from build123d import *

# Parameters (mm, degrees)
BOSS_EXTRUDE1_DEPTH = 0.8
SKETCH2_W           = 0.45
SKETCH2_H           = 25.2222
BOSS_EXTRUDE2_DEPTH = 9.525


with BuildPart() as part:
    # Sketch1 → Boss-Extrude1 (new body)
    with BuildSketch(Plane.XY):
        Polygon((0, 0), (0, 25.2222), (6.1722, 25.2222), (6.1722, 15.6972), (15.6972, 15.6972), (15.6972, 9.525), (6.1722, 9.525), (6.1722, 0), align=None)
    extrude(amount=BOSS_EXTRUDE1_DEPTH)

    # Sketch2 → Boss-Extrude2 (add)
    with BuildSketch(Plane.XY.offset(0.8)):
        Polygon((6.1722, 0), (6.1722, 9.525), (15.6972, 9.525), (15.6972, 9.975), (5.7222, 9.975), (5.7222, 0), align=None)
        Polygon((15.6972, 15.6972), (6.1722, 15.6972), (6.1722, 25.2222), (5.7222, 25.2222), (5.7222, 15.2472), (15.6972, 15.2472), align=None)
        with Locations((0.225, 12.6111)):
            Rectangle(SKETCH2_W, SKETCH2_H)
    extrude(amount=BOSS_EXTRUDE2_DEPTH)


solid = part.part
The model under review builds one solid part; all positions refer to its coordinate system, in mm. A direction names the side the tool comes from. Round coordinates to 2 decimals unless told otherwise and drop trailing zeros. Loops run counter-clockwise (first coordinate to the right, second up) from the corner with the lowest first, then second, coordinate; pieces in that order, holes last. Notation, with made-up numbers: M -14.75,-31 L 30.25,-31 A28 cw 30.25,2 Z; hole C 38,74.25 d10. An arc over 180 degrees is marked long. Answer as CSV lines item,"result". Start each with the question number.
Item 1: Insertion check: P1, Ø4, axis at x = 12.5, z = 6.5, coming from the -Y side (3 decimals); P2, Ø1.5, axis at x = 11, z = 5, coming from the +Y side; P3, Ø2, axis at y = 4.5, z = 2, coming from the +X side; P4, Ø1, axis at x = 7, y = 3.5, coming from the +Z side. Each pin has a flat end and moves straight along its axis. Give the tip position at first contact, or say it passes through.
Item 2: Wall thickness on line 1 (X direction, y = 2, z = 6.25); line 2 (Y direction, x = 8, z = 1.5) (3 decimals); line 3 (X direction, y = 14, z = 1.25): over which ranges is each line inside the solid? List them lowest first. Write a range as [from, to].
Item 3: Consider section C-C (x = 10.5). Write out the cut boundary in (y, z) (3 decimals).
Item 4: For faces 5 (the face through (11, 15.697, 5)), 6 (the face through (11, 9.975, 5)), 7 (the face through (11, 9.525, 5)), 8 (the face through (5.722, 20, 5)), list the 3-axis set-ups (+Z, -Z, +X, -X, +Y, -Y) from which the entire face can be reached by the end or side of a thin tool; tool diameter is ignored.
Item 5: Consider section B-B (y = 21.75). Write out the cut boundary in (x, z) (3 decimals), then the cut area to 3 significant figures.
Item 6: Consider section A-A (z = 1.5). Write out the cut boundary in (x, y) (3 decimals).
Item 7: Consider section D-D (y = 10.5). Write out the cut boundary in (x, z) (3 decimals), then the cut area to 3 significant figures.
Item 8: Mouldability with a two-part tool opening along X and no side actions: class faces 1 (the face through (6.172, 5, 5)), 2 (the face through (0.3, 0, 3.6)), 3 (the face through (0.45, 12, 5)), 4 (the face through (5, 13, 0.8)) as released by +X, released by -X, zero draft, split by the parting line, or undercut.
Answer:
1,P1,"stops at y = 9.525"
1,P2,"stops at y = 15.7"
1,P3,"stops at x = 6.17"
1,P4,"passes through"
2,line 1,"x = [0, 0.45], [5.72, 6.17]"
2,line 2,"y = [9.525, 9.975], [15.247, 15.697]"
2,line 3,"x = [0, 0.45]"
3,outline,"M 9.525,0 L 15.697,0 L 15.697,10.325 L 15.247,10.325 L 15.247,0.8 L 9.975,0.8 L 9.975,10.325 L 9.525,10.325 Z"
4,face 5,"+Z, -Z, +X, +Y"
4,face 6,"+Z, +X"
4,face 7,"+Z, -Z, +X, -Y"
4,face 8,"+Z, +Y, -Y"
5,outline,"M 0,0 L 6.172,0 L 6.172,10.325 L 5.722,10.325 L 5.722,0.8 L 0.45,0.8 L 0.45,10.325 L 0,10.325 Z"
5,area,"13.5 mm^2"
6,outline,"M 0,0 L 0.45,0 L 0.45,25.222 L 0,25.222 Z; M 5.722,0 L 6.172,0 L 6.172,9.525 L 15.697,9.525 L 15.697,9.975 L 5.722,9.975 Z; M 5.722,15.247 L 15.697,15.247 L 15.697,15.697 L 6.172,15.697 L 6.172,25.222 L 5.722,25.222 Z"
7,outline,"M 0,0 L 15.697,0 L 15.697,0.8 L 0.45,0.8 L 0.45,10.325 L 0,10.325 Z"
7,area,"16.8 mm^2"
8,face 1,"released by +X"
8,face 2,"zero draft"
8,face 3,"undercut"
8,face 4,"undercut"
